Work out the finished part from the listing and answer in its coordinate system (mm). Face numbers are marked on the shaded views. A direction names the side the tool comes from. Give positions to 0.01 mm unless a question says otherwise; leave off trailing zeros. Order: outer loops, then holes, each group sorted by start corner. A loop starts at its lowest first (then second) coordinate and runs counter-clockwise, first axis right, second up. Notation, with made-up numbers: (71.25, 6) - (98.25, 6) arc R25 cw to (98.25, 32) - close; hole circle Ø4 at (-31, 24.25). An arc over 180 degrees is marked (long way). Write each question's results on one line, items separated by ' | '.
from build123d import *

# Parameters (mm, degrees)
SKETCH1_R           = 1
BOSS_EXTRUDE1_DEPTH = 2.5
SKETCH2_R           = 4.5
SKETCH2_R_2         = 3
BOSS_EXTRUDE2_DEPTH = 2
SKETCH3_R           = 1.5
CUT_EXTRUDE1_DEPTH  = 3.5
SKETCH4_R           = 3.5
CUT_EXTRUDE2_DEPTH  = 0.2


with BuildPart() as part:
    # Sketch1 → Boss-Extrude1 (new body)
    with BuildSketch(Plane(origin=(0, 0, 0), x_dir=(1, 0, 0), z_dir=(0, 1, 0))):
        with BuildLine():
            Line((0.208333333, 2.491304321), (-29.583333333, 4.982608643))
            ThreePointArc((-29.583333333, 4.982608643), (-35, 0), (-29.583333333, -4.982608643))
            Line((-29.583333333, -4.982608643), (0.208333333, -2.491304321))
            ThreePointArc((0.208333333, -2.491304321), (2.5, 0), (0.208333333, 2.491304321))
        make_face()
        with Locations((-15, 0)):
            Circle(SKETCH1_R, mode=Mode.SUBTRACT)
        with Locations((-10, 0)):
            Circle(SKETCH1_R, mode=Mode.SUBTRACT)
        with Locations((-5, 0)):
            Circle(SKETCH1_R, mode=Mode.SUBTRACT)
        Circle(SKETCH1_R, mode=Mode.SUBTRACT)
    extrude(amount=BOSS_EXTRUDE1_DEPTH)

    # Sketch2 → Boss-Extrude2 (add)
    with BuildSketch(Plane(origin=(0, 2.5, 0), x_dir=(1, 0, 0), z_dir=(0, 1, 0))):
        with Locations((-30, 0)):
            Circle(SKETCH2_R)
        with Locations((-30, 0)):
            Circle(SKETCH2_R_2, mode=Mode.SUBTRACT)
    extrude(amount=BOSS_EXTRUDE2_DEPTH)

    # Sketch3 → Cut-Extrude1 (cut, through all)
    with BuildSketch(Plane(origin=(0, 2.5, 0), x_dir=(1, 0, 0), z_dir=(0, 1, 0))):
        with Locations((-30, 0)):
            Circle(SKETCH3_R)
    extrude(amount=-CUT_EXTRUDE1_DEPTH, mode=Mode.SUBTRACT)

    # Sketch4 → Cut-Extrude2 (cut)
    with BuildSketch(Plane.XZ):
        with Locations((-30, 0)):
            Circle(SKETCH4_R)
    extrude(amount=-CUT_EXTRUDE2_DEPTH, mode=Mode.SUBTRACT)


solid = part.part
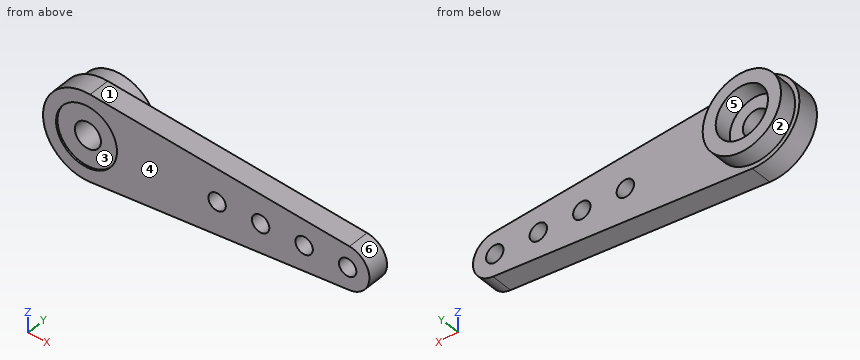
1. A tool of negligible diameter and unlimited length cuts with its end or side. For the marked faces 5 and 6, from which of +Z, -Z, +X, -X, +Y, -Y can it reach the whole face along a straight path? Write none if from no direction.
Answer list:
face 5: +Y | face 6: +X, +Y, -Y
2. Determine the mould class of the marked faces 1, 2, 3 and 4 for opening direction Z: +Z half, -Z half, draft (parallel to the pull), parting line (faces both ways), or undercut.
Answer list:
face 1: +Z half | face 2: parting line | face 3: undercut | face 4: draft
3. A cutting plane is placed at B-B, the plane x = -5. Write down the section's boundary in (y, z), then the cut area to 3 significant figures.
Answer list:
outline: (0, -2.93) - (2.5, -2.93) - (2.5, -1) - (0, -1) - close; (0, 1) - (2.5, 1) - (2.5, 2.93) - (0, 2.93) - close | area: 9.63 mm^2
4. A cutting plane is placed at D-D, the plane z = -4. Write down the section's boundary in (x, y).
Answer list:
outline: (-33, 0) - (-17.83, 0) - (-17.83, 2.5) - (-27.94, 2.5) - (-27.94, 4.5) - (-32.06, 4.5) - (-32.06, 2.5) - (-33, 2.5) - close
5. A cutting plane is placed at C-C, the plane z = 0. State how many separate pieces and enclosed holes the cut face has, then the cut area to 4 significant figures.
Answer list:
separate pieces: 6 | enclosed holes: 0 | area: 71.45 mm^2
6. Straight lines are drawn through the part: line 1 (X direction, y = 0.8, z = 0); line 2 (X direction, y = 3.05, z = 0); line 3 (Z direction, x = -30, y = 3.25). For each, find the intervals that lie inside material, in ascending order. Write a range as [from, to].
Answer list:
line 1: [-35, -31.5], [-28.5, -16], [-14, -11], [-9, -6], [-4, -1], [1, 2.5] | line 2: [-34.5, -33], [-27, -25.5] | line 3: [-4.5, -3], [3, 4.5]
7. A cutting plane is placed at A-A, the plane y = 1.5. Write down the section's boundary in (x, z), then the cut area to 3 significant figures.
Answer list:
outline: (-29.58, -4.98) - (0.21, -2.49) arc R2.5 ccw to (0.21, 2.49) - (-29.58, 4.98) arc R5 ccw (long way) to start; hole circle Ø3 at (-30, 0); hole circle Ø2 at (-15, 0); hole circle Ø2 at (-10, 0); hole circle Ø2 at (-5, 0); hole circle Ø2 at (0, 0) | area: 255 mm^2
8. Given P1, Ø1.5, axis at x = -3, y = 2, coming from the +Z side; P2, Ø1.8, axis at x = -30, z = 0, coming from the -Y side; P3, Ø4, axis at x = -30, z = 0, coming from the -Y side; P4, Ø3, axis at x = -22.5, z = -0.5, coming from the +Y side, each flat-ended and moving along its own axis, determine where each tip first touches the part or whether it passes through.
Answer list:
P1: z = 2.82 | P2: through | P3: y = 0.2 | P4: y = 2.5
